```python
from build123d import *

# Parameters (mm, degrees)
ESQUISSE1_W             = 380
ESQUISSE1_H             = 150
BOSS_EXTRU_1_DEPTH      = 20
ESQUISSE2_R             = 50
ESQUISSE2_W             = 36.086047363
ESQUISSE2_H             = 20
ENL_V_MAT_EXTRU_2_DEPTH = 21
ESQUISSE4_R             = 67.75
ENL_V_MAT_EXTRU_3_DEPTH = 10
ENL_V_MAT_EXTRU_4_DEPTH = 21


with BuildPart() as part:
    # Esquisse1 → Boss.-Extru.1 (new body)
    with BuildSketch(Plane(origin=(0, 0, 0), x_dir=(1, 0, 0), z_dir=(0, 1, 0))):
        Rectangle(ESQUISSE1_W, ESQUISSE1_H)
    extrude(amount=BOSS_EXTRU_1_DEPTH)

    # Esquisse2 → Enlèv. mat.-Extru.2 (cut, through all)
    with BuildSketch(Plane(origin=(0, 0, 0), x_dir=(-1, 0, 0), z_dir=(0, -1, 0))):
        with BuildLine():
            Line((172.912878475, -10), (190, -10))
            Line((190, -10), (190, 10))
            Line((190, 10), (172.912878475, 10))
            ThreePointArc((172.912878475, 10), (174.472657823, 5.107741092), (175, 0))
            ThreePointArc((175, 0), (174.472657823, -5.107741092), (172.912878475, -10))
        make_face()
        with BuildLine():
            ThreePointArc((172.912878475, 10), (125, 0), (172.912878475, -10))
            Line((172.912878475, -10), (159.255580532, -10))
            Line((159.255580532, -10), (159.255580532, 10))
            Line((159.255580532, 10), (172.912878475, 10))
        make_face()
        with BuildLine():
            Line((159.255580532, -10), (172.912878475, -10))
            ThreePointArc((172.912878475, -10), (174.472657823, -5.107741092), (175, 0))
            ThreePointArc((175, 0), (174.472657823, 5.107741092), (172.912878475, 10))
            Line((172.912878475, 10), (159.255580532, 10))
            Line((159.255580532, 10), (159.255580532, -10))
        make_face()
        Circle(ESQUISSE2_R)
        with BuildLine():
            Line((-154.989806054, 10), (-154.989806054, -10))
            Line((-154.989806054, -10), (-172.912878475, -10))
            ThreePointArc((-172.912878475, -10), (-144.892258908, -24.472657823), (-125, 0))
            ThreePointArc((-125, 0), (-144.892258908, 24.472657823), (-172.912878475, 10))
            Line((-172.912878475, 10), (-154.989806054, 10))
        make_face()
        with BuildLine():
            Line((-172.912878475, -10), (-154.989806054, -10))
            Line((-154.989806054, -10), (-154.989806054, 10))
            Line((-154.989806054, 10), (-172.912878475, 10))
            ThreePointArc((-172.912878475, 10), (-175, 0), (-172.912878475, -10))
        make_face()
        with Locations((-208.043023682, 0)):
            Rectangle(ESQUISSE2_W, ESQUISSE2_H)
        with BuildLine():
            Line((-190, -10), (-172.912878475, -10))
            ThreePointArc((-172.912878475, -10), (-175, 0), (-172.912878475, 10))
            Line((-172.912878475, 10), (-190, 10))
            Line((-190, 10), (-190, -10))
        make_face()
    extrude(amount=-ENL_V_MAT_EXTRU_2_DEPTH, mode=Mode.SUBTRACT)

    # Esquisse4 → Enlèv. mat.-Extru.3 (cut)
    with BuildSketch(Plane(origin=(0, 20, 0), x_dir=(1, 0, 0), z_dir=(0, 1, 0))):
        Circle(ESQUISSE4_R)
    extrude(amount=-ENL_V_MAT_EXTRU_3_DEPTH, mode=Mode.SUBTRACT)

    # Esquisse5 → Enlèv. mat.-Extru.4 (cut, through all)
    with BuildSketch(Plane(origin=(0, 20, 0), x_dir=(1, 0, 0), z_dir=(0, 1, 0))):
        with BuildLine():
            ThreePointArc((-45.987048839, -59.246867758), (-92.825023805, -43.159932782), (-142.192482618, -39.230634361))
            ThreePointArc((-142.192482618, -39.230634361), (-171.275688102, -33.87248287), (-188.729833462, -10))
            Line((-188.729833462, -10), (-190, -10))
            Line((-190, -10), (-190, -75))
            Line((-190, -75), (-6.82e-07, -75))
            ThreePointArc((-6.82e-07, -75), (-24.305194399, -70.952501896), (-45.987048839, -59.246867758))
        make_face()
        with BuildLine():
            ThreePointArc((-188.729833462, 10), (-171.275688102, 33.87248287), (-142.192482618, 39.230634361))
            ThreePointArc((-142.192482618, 39.230634361), (-92.140738349, 39.871003351), (-45.987048839, 59.246867758))
            ThreePointArc((-45.987048839, 59.246867758), (-24.305194053, 70.952502014), (4.9e-08, 75))
            Line((4.9e-08, 75), (-190, 75))
            Line((-190, 75), (-190, 10))
            Line((-190, 10), (-188.729833462, 10))
        make_face()
        with BuildLine():
            Line((190, 75), (4.9e-08, 75))
            ThreePointArc((4.9e-08, 75), (24.3051941, 70.952501998), (45.987048839, 59.246867758))
            ThreePointArc((45.987048839, 59.246867758), (90.245637387, 41.772491768), (137.68369163, 38.056649198))
            ThreePointArc((137.68369163, 38.056649198), (169.266874889, 35.054065841), (188.729833462, 10))
            Line((188.729833462, 10), (190, 10))
            Line((190, 10), (190, 75))
        make_face()
        with BuildLine():
            ThreePointArc((45.671882044, -59.490160452), (24.116777718, -71.016765855), (-6.82e-07, -75))
            Line((-6.82e-07, -75), (190, -75))
            Line((190, -75), (190, -10))
            Line((190, -10), (188.729833462, -10))
            ThreePointArc((188.729833462, -10), (170.810992049, -34.159956234), (141.123685996, -39.002705671))
            ThreePointArc((141.123685996, -39.002705671), (91.61350334, -40.933403872), (45.671882044, -59.490160452))
        make_face()
    extrude(amount=-ENL_V_MAT_EXTRU_4_DEPTH, mode=Mode.SUBTRACT)


solid = part.part
```
The model under review builds one solid part; all positions refer to its coordinate system, in mm. A direction names the side the tool comes from. Round coordinates to 2 decimals unless told otherwise and drop trailing zeros. Loops run counter-clockwise (first coordinate to the right, second up) from the corner with the lowest first, then second, coordinate; pieces in that order, holes last. Notation, with made-up numbers: M -39.75,68 L -33.75,68 A35 cw -33.75,104 Z; hole C 41,43.5 d3. An arc over 180 degrees is marked long. Write item = value, one per line.
Item 1: Take a section at D-D on x = 22. Write out the cut boundary in (y, z), then the cut area to 3 significant figures.
Return value:
outline = M 0,-71.7 L 20,-71.7 L 20,-64.08 L 10,-64.08 L 10,-44.9 L 0,-44.9 Z; M 0,44.9 L 10,44.9 L 10,64.08 L 20,64.08 L 20,71.7 L 0,71.7 Z
area = 688 mm2
Item 2: Machinability: for faces 5 (the flat face through (-14.9, 20, 66.3)), 6 (the cylindrical face through (-92.145, 10.14, 43.303)), 7 (the flat face through (-181, 10, 10)), 8 (the cylindrical face through (89.594, 10.14, -41.924)), 9 (the flat face through (-5, 10, 50)), which of the approach directions +Z, -Z, +X, -X, +Y, -Y give a long, thin tool a straight path to every point of the face, cutting with its end or side? Answer none if there is none.
Return value:
face_5 = +Z, -Z, +X, -X, +Y
face_6 = +Z, +Y, -Y
face_7 = -X, +Y, -Y
face_8 = -Z, +Y, -Y
face_9 = +Y
Item 3: Take a section at C-C on z = -29. Write out the cut boundary in (x, y), then the cut area to 3 significant figures.
Return value:
outline = M -177.55,0 L -40.73,0 L -40.73,10 L -61.23,10 L -61.23,20 L -177.55,20 Z; M 40.73,0 L 177.55,0 L 177.55,20 L 61.23,20 L 61.23,10 L 40.73,10 Z
area = 5,060 mm2
Item 4: Insertion check: P1, Ø8, axis at x = 114.5, y = 5.5, coming from the +Z side; P2, Ø4, axis at x = -48.5, y = 9.5, coming from the -Z side; P3, Ø4.5, axis at x = 178.5, y = 7, coming from the -Z side. Each pin has a flat end and moves straight along its axis. Give the tip position at first contact, or say it passes through.
Return value:
P1 = 38.17
P2 = -58.91
P3 = -30.18
Item 5: Take a section at A-A on x = 160.5. Write out the cut boundary in (y, z), then the cut area to 3 significant figures.
Return value:
outline = M 0,-38.6 L 20,-38.6 L 20,-22.69 L 0,-22.69 Z; M 0,22.69 L 20,22.69 L 20,38.6 L 0,38.6 Z
area = 636 mm2
Item 6: Take a section at B-B on y = 4. Write out the cut boundary in (x, z), then the cut area to 3 significant figures.
Return value:
outline = M -188.73,-10 A40 ccw -142.19,-39.23 A130.93 cw -45.99,-59.25 A75 ccw 45.99,-59.25 A160.34 cw 137.68,-38.06 A40 ccw 188.73,-10 L 172.91,-10 A25 cw long 172.91,10 L 188.73,10 A40 ccw 141.12,39 A144.37 cw 45.67,59.49 A75 ccw -45.99,59.25 A197.5 cw -142.19,39.23 A40 ccw -188.73,10 L -172.91,10 A25 cw long -172.91,-10 Z; hole C 0,0 d100
area = 23,500 mm2
Item 7: The part is to be moulded in two halves that separate along Z. For faces 1 (the flat face through (181, 10, -10)), 2 (the flat face through (181, 10, 10)), 3 (the cylindrical face through (-92.83, 10.14, -39.73)), 4 (the cylindrical face through (171.178, 10.14, 33.933)), say which applies: released by +Z, released by -Z, zero draft, split by the parting line, or undercut.
Return value:
face_1 = undercut
face_2 = undercut
face_3 = released by -Z
face_4 = released by +Z
Item 8: For line 1 (X direction, y = 10.75, z = 0); line 2 (X direction, y = 18.25, z = -12); line 3 (X direction, y = 4, z = 17), list the stretches that pass through material, from the lowest coordinate up. Write a range as [from, to].
Return value:
line_1 = [-125, -67.75], [67.75, 125]
line_2 = [-188.16, -171.93], [-128.07, -66.68], [66.68, 128.07], [171.93, 188.16]
line_3 = [-186.21, -168.33], [-131.67, -47.02], [47.02, 131.67], [168.33, 186.21]
